Here's how the part is built. I have some questions about the finished solid (model axes, mm). Face numbers are marked on the shaded views. A direction names the side the tool comes from. Round coordinates to 2 decimals unless told otherwise and drop trailing zeros. Loops run counter-clockwise (first coordinate to the right, second up) from the corner with the lowest first, then second, coordinate; pieces in that order, holes last. Notation, with made-up numbers: (46, 59) -> (98, 59) arc R29 cw to (98, 95) -> close; hole circle Ø5 at (-23.75, 5.5). An arc over 180 degrees is marked (long way). Use one line per item in the form item = value. Start each with the question number.
Item 1: If we section it at A-A (z = -10.5): Write out the boundary of the cut face in (x, y), then the cut area to 3 significant figures.
Item 2: If we section it at D-D (x = 11): Write out the boundary of the cut face in (y, z).
Item 3: For the marked faces 4, 5, 6 and 7, which set-ups out of +Z, -Z, +X, -X, +Y, -Y let a thin tool reach every point of the face, with its end or its side?
Item 4: I'm going to push flat-ended pins straight in: pin 1 Ø8 at (y, z) = (-12.5, 6) entering from -X; pin 2 Ø2.5 at (x, y) = (11, -2) entering from +Z; pin 3 Ø2.5 at (x, z) = (15, -16.5) entering from +Y; pin 4 Ø4 at (x, y) = (15.5, -1) entering from -Z. Where does each tip first touch, or does it pass through?
Item 5: If I drill on L1, parallel to Z at x = 7.65, y = 7.25; L2, parallel to Y at x = 14, z = 0; L3, parallel to Y at x = 5.25, z = 0, over which ranges is the centre line in solid material (lowest first)? Write a range as [from, to].
Item 6: Thinking about a two-plate mould opening in Y: for the marked faces 1, 2 and 3, which applies, released by +Y, released by -Y, zero draft, split by the parting line, or undercut?
Item 7: If we section it at C-C (y = -7.25): Write out the boundary of the cut face in (x, z).
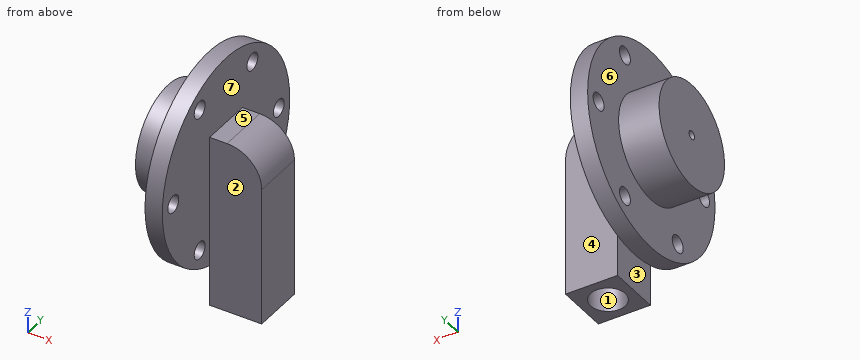
Autodesk Inventor part; units mm, degrees
ref_plane "Work Plane1" through (0, 0, -7.5) normal (0, 0, 1) x (1, 0, 0)
ref_plane "YZ Plane" through (0, 0, 0) normal (1, 0, 0) x (0, 1, 0)
ref_plane "XZ Plane" through (0, 0, 0) normal (0, 1, 0) x (-1, 0, 0)
sketch "Sketch1" plane through (0, 0, 0) normal (0, 0, 1) x (1, 0, 0)
  line L0 (0, 0) -> (0, 9)
  line L1 (0, 9) -> (7, 9)
  line L2 (7, 9) -> (7, 17.5)
  line L3 (7, 17.5) -> (10, 17.5)
  line L4 (10, 17.5) -> (10, 0)
  line L5 (10, 0) -> (0, 0)
  dimension "d0" = 18
  dimension "d1" = 35
  dimension "d2" = 7
  dimension "d3" = 3
revolve "Revolution1" add sketch "Sketch1" angle 360 about axis through (10, 0, 0) along (-1, 0, 0)
sketch "Sketch2" plane through (0, 0, 0) normal (0, 1, 0) x (-1, 0, 0)
  line L0 (-10, -17.5) -> (-10, 17.5)
  line L1 (-10, 6) -> (-13, 6)
  line L2 (-19, 0) -> (-19, -24)
  line L3 (-19, -24) -> (-10, -24)
  line L4 (-10, -24) -> (-10, 6)
  line L5 (-10, -17.5) -> (-7, -17.5)
  arc A0 (-13, 6) -> (-19, 0) centre (-13, 0) ccw
  point P0 (0, 0)
  point P1 (-8.5, -17.5)
  dimension "d6" = 30
  dimension "d7" = 9
  dimension "d8" = 6.5
  dimension "d9" = 6
extrude "Extrusion1" add sketch "Sketch2" along normal mid plane 9
sketch "Sketch3" plane through (19, 4.5, -24) normal (0, 0, -1) x (-1, 0, 0)
  line L0 (9, 0) -> (9, -9)
  line L1 (0, 0) -> (9, 0)
  point P0 (19, -4.5)
  point P1 (4.5, -4.5)
  point P2 (9, -4.5)
  dimension "d19" = 4.5
  dimension "d20" = 4.5
hole "Hole1" at (14.5, 0, -24) direction (0, 0, 1) diameter 4.917 depth 18 counterbore diameter 6 counterbore depth 7
ref_plane "Work Plane1" through (0, 0, -7.5) normal (0, 0, 1) x (1, 0, 0)
sketch "Sketch4" plane through (0, 0, -7.5) normal (0, 0, 1) x (1, 0, 0)
  circle A0 centre (14.5, 0) radius 3
  point P0 (0, 0)
hole "Hole2" at (14.5, 0, -7.5) direction (0, 0, 1) diameter 1.5 depth 7.5
sketch "Sketch5" plane through (10, 0, 0) normal (1, 0, 0) x (0, 0, -1)
  line L0 (-6, 4.5) -> (16.9115, 4.5)
  arc A0 (16.9115, 4.5) -> (16.9115, -4.5) centre (0, 0) ccw
  line L1 (16.9115, -4.5) -> (-6, -4.5)
  line L2 (-6, -4.5) -> (-6, 4.5)
  circle A1 centre (0, 0) radius 14.5 construction
  line L3 (0, -4.5) -> (0, 4.5)
  line L4 (0, 0) -> (12.5574, 7.25) construction
  line L5 (0, 0) -> (27.6817, 0) construction
  dimension "d29" = 29
  dimension "d30" = 30
hole "Hole3" at (10, 7.25, -12.5574) direction (-1, 0, 0) diameter 3 depth 3
pattern_circular "Circular Pattern1" count 6 over 360 about axis through (8.5, 0, 0) along (-1, 0, 0) of "Hole3"
sketch "Sketch6" plane through (0, 0, 0) normal (-1, 0, 0) x (0, 0, 1)
  circle A0 centre (0, 0) radius 9
hole "Hole4" at (0, 0, 0) direction (1, 0, 0) diameter 1.5 depth 14.5
properties part number "155 part 1" material "Gold"
Values found:
q1.outline = (7, -14) -> (10, -14) -> (10, -4.5) -> (19, -4.5) -> (19, 4.5) -> (10, 4.5) -> (10, 14) -> (7, 14) -> close; hole circle Ø4.92 at (14.5, 0)
q1.area = 146 mm2
q2.outline = (-4.5, -24) -> (4.5, -24) -> (4.5, 6) -> (-4.5, 6) -> close; hole circle Ø1.5 at (0, 0)
q3.face_4 = +Z, -Z, +X, +Y
q3.face_5 = +Z, +X, +Y, -Y
q3.face_6 = -X
q3.face_7 = +Z, +X
q4.pin_1 = 7
q4.pin_2 = 17.46
q4.pin_3 = 4.5
q4.pin_4 = -24
q5.L1 = [-15.93, -14.06], [-11.06, 11.06], [14.06, 15.93]
q5.L2 = [-4.5, -0.75], [0.75, 4.5]
q5.L3 = [-9, -0.75], [0.75, 9]
q6.face_1 = undercut
q6.face_2 = released by -Y
q6.face_3 = zero draft
q7.outline = (0, -5.33) -> (7, -5.33) -> (7, -11.06) -> (10, -11.06) -> (10, 11.06) -> (7, 11.06) -> (7, 5.33) -> (0, 5.33) -> close; (7, -15.93) -> (10, -15.93) -> (10, -14.06) -> (7, -14.06) -> close; (7, 14.06) -> (10, 14.06) -> (10, 15.93) -> (7, 15.93) -> close
